Here's how the part is built. I have some questions about the finished solid (model axes, mm). Face numbers are marked on the shaded views. A direction names the side the tool comes from. Give positions to 0.01 mm unless a question says otherwise; leave off trailing zeros. Write each loop counter-clockwise with the first axis right and the second up, starting at its lowest first coordinate (ties: lowest second). Pieces come first, ordered by that corner, then holes. Notation, with made-up numbers: (42.25, -35.75) - (87.25, -35.75) arc R22 cw to (87.25, -7.75) - close; hole circle Ø2 at (-24.5, 45). An arc over 180 degrees is marked (long way). Use a Markdown table: item, result.
```python
from build123d import *

# Parameters (mm, degrees)
SKETCH1_W           = 60
SKETCH1_H           = 46
SKETCH1_W_2         = 50
SKETCH1_H_2         = 36
BOSS_EXTRUDE1_DEPTH = 10.5
SKETCH2_W           = 50
SKETCH2_H           = 36
BOSS_EXTRUDE2_DEPTH = 1.6
FILLET1_R           = 3
SKETCH3_R           = 1.4
BOSS_EXTRUDE3_DEPTH = 5
CHAMFER1_SIZE       = 0.35
CHAMFER2_SIZE       = 0.5


with BuildPart() as part:
    # Sketch1 → Boss-Extrude1 (new body)
    with BuildSketch(Plane(origin=(0, 0, 0), x_dir=(1, 0, 0), z_dir=(0, 1, 0))):
        with Locations((25, 18)):
            Rectangle(SKETCH1_W, SKETCH1_H)
        with Locations((25, 18)):
            Rectangle(SKETCH1_W_2, SKETCH1_H_2, mode=Mode.SUBTRACT)
    extrude(amount=BOSS_EXTRUDE1_DEPTH)

    # Sketch2 → Boss-Extrude2 (add)
    with BuildSketch(Plane(origin=(0, 0, 0), x_dir=(1, 0, 0), z_dir=(0, 1, 0))):
        with Locations((25, 18)):
            Rectangle(SKETCH2_W, SKETCH2_H)
    extrude(amount=BOSS_EXTRUDE2_DEPTH)

    # Fillet1
    fillet1_edges = [part.edges().sort_by_distance(p)[0] for p in [
        (-5, 5.25, -41),
        (55, 5.25, -41),
        (55, 5.25, 5),
        (-5, 5.25, 5),
    ]]
    fillet(fillet1_edges, radius=FILLET1_R)

    # Sketch3 → Boss-Extrude3 (add)
    with BuildSketch(Plane(origin=(0, 10.5, 0), x_dir=(1, 0, 0), z_dir=(0, 1, 0))):
        with Locations((25, 38.5)):
            Circle(SKETCH3_R)
        with Locations((-2.5, 18)):
            Circle(SKETCH3_R)
        with Locations((25, -2.5)):
            Circle(SKETCH3_R)
    extrude(amount=BOSS_EXTRUDE3_DEPTH)

    # Chamfer1
    chamfer1_edges = [part.edges().sort_by_distance(p)[0] for p in [
        (23.6, 15.5, -38.5),
        (-3.9, 15.5, -18),
        (23.6, 15.5, 2.5),
    ]]
    chamfer(chamfer1_edges, length=CHAMFER1_SIZE)

    # Chamfer2
    chamfer2_edges = [part.edges().sort_by_distance(p)[0] for p in [
        (25, 0, -41),
        (-5, 0, -18),
        (55, 0, -18),
        (25, 0, 5),
        (-4.121320344, 0, 4.121320344),
        (54.121320344, 0, 4.121320344),
        (-4.121320344, 0, -40.121320344),
        (54.121320344, 0, -40.121320344),
    ]]
    chamfer(chamfer2_edges, length=CHAMFER2_SIZE)


solid = part.part
```
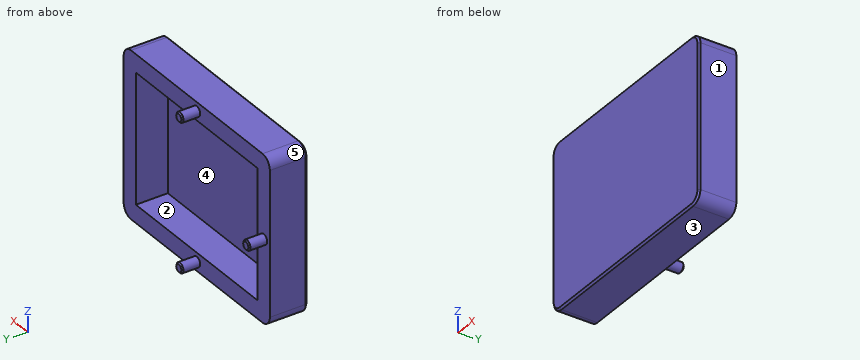
Item 1: I need wall thicknesses on line 1 along Z through (x, y) = (21, 6); line 2 along X through (y, z) = (4.5, -3.5); line 3 along Y through (x, z) = (22.5, -35.5). Which ranges of each line are inside material? Lowest first, please. Write a range as [from, to].
Values:
| item | result |
|---|---|
| line 1 | z = [-41, -36], [0, 5] |
| line 2 | x = [-5, 0], [50, 55] |
| line 3 | y = [0, 1.6] |
Item 2: Will these pins go through, and if not, where does the flat tip stop? pin 1 Ø23 at (x, z) = (30, -11) entering from +Y; pin 2 Ø10 at (x, z) = (17.5, -10) entering from +Y.
Values:
| item | result |
|---|---|
| pin 1 | stops at y = 10.5 |
| pin 2 | stops at y = 1.6 |
Item 3: If we section it at A-A, the plane y = 6.75: Write out the boundary of the cut face in (x, z), plus the area to 3 significant figures.
Values:
| item | result |
|---|---|
| outline | (-5, -38) arc R3 ccw to (-2, -41) - (52, -41) arc R3 ccw to (55, -38) - (55, 2) arc R3 ccw to (52, 5) - (-2, 5) arc R3 ccw to (-5, 2) - close; hole (0, -36) - (50, -36) - (50, 0) - (0, 0) - close |
| area | 952 mm2 |
Item 4: For the marked faces 4 and 5, which set-ups out of +Z, -Z, +X, -X, +Y, -Y let a thin tool reach every point of the face, with its end or its side?
Values:
| item | result |
|---|---|
| face 4 | +Y |
| face 5 | +Z, -X, +Y, -Y |
Item 5: Thinking about a two-plate mould opening in X: for the marked faces 1, 2 and 3, which applies, +X half, -X half, draft (parallel to the pull), parting line (faces both ways), or undercut?
Values:
| item | result |
|---|---|
| face 1 | +X half |
| face 2 | undercut |
| face 3 | draft |
Item 6: If we section it at C-C, the plane x = 25: Write out the boundary of the cut face in (y, z), plus the area to 3 significant figures.
Values:
| item | result |
|---|---|
| outline | (0, -40.5) - (0.5, -41) - (10.5, -41) - (10.5, -39.9) - (15.15, -39.9) - (15.5, -39.55) - (15.5, -37.45) - (15.15, -37.1) - (10.5, -37.1) - (10.5, -36) - (1.6, -36) - (1.6, 0) - (10.5, 0) - (10.5, 1.1) - (15.15, 1.1) - (15.5, 1.45) - (15.5, 3.55) - (15.15, 3.9) - (10.5, 3.9) - (10.5, 5) - (0.5, 5) - (0, 4.5) - close |
| area | 190 mm2 |
Item 7: If we section it at B-B, the plane z = -18: Write out the boundary of the cut face in (x, y), plus the area to 3 significant figures.
Values:
| item | result |
|---|---|
| outline | (-5, 0.5) - (-4.5, 0) - (54.5, 0) - (55, 0.5) - (55, 10.5) - (50, 10.5) - (50, 1.6) - (0, 1.6) - (0, 10.5) - (-1.1, 10.5) - (-1.1, 15.15) - (-1.45, 15.5) - (-3.55, 15.5) - (-3.9, 15.15) - (-3.9, 10.5) - (-5, 10.5) - close |
| area | 199 mm2 |
Item 8: If we section it at D-D, the plane y = 11.75: Write out the boundary of the cut face in (x, z), plus the area to 3 significant figures.
Values:
| item | result |
|---|---|
| outline | circle Ø2.8 at (-2.5, -18); circle Ø2.8 at (25, -38.5); circle Ø2.8 at (25, 2.5) |
| area | 18.5 mm2 |
